Check sheet for the modelled part. Datum: model origin and axes. Units: mm. Face numbers are marked on the shaded views. A direction names the side the tool comes from. Coordinates: 2 decimals unless noted, no trailing zeros. Write each loop counter-clockwise with the first axis right and the second up, starting at its lowest first coordinate (ties: lowest second). Pieces come first, ordered by that corner, then holes. Notation, with made-up numbers: M 82,-30 L 115,-30 A25 cw 115,-17 Z; hole C 24,8 d7. An arc over 180 degrees is marked long. Answer as CSV lines item,"result".
from build123d import *

# Parameters (mm, degrees)
EXTRUDE1_DEPTH      = 3.9
EXTRUDE1_DEPTH_BACK = 3.9
SKETCH2_W           = 4.5
SKETCH2_H           = 25.2
SKETCH2_W_2         = 29.65
SKETCH2_H_2         = 5.85
EXTRUDE2_DEPTH      = 3.5
CHAMFER1_SIZE       = 3
CHAMFER1_SIZE2      = 3.451105222
CHAMFER2_SIZE       = 2
CHAMFER2_SIZE2      = 3.464101615
CHAMFER3_SIZE       = 1
EXTRUDE3_REACH      = 40.849
SKETCH4_R           = 3
FILLET1_R           = 0.8
EXTRUDE4_REACH      = 40.849
SKETCH5_R           = 3


# Read off the part's stored shape, not the designer's step: Mirror1
with BuildPart() as part:
    # Sketch1 → Extrude1 (new, two sides: drawn at the far end of the back side and taken through both)
    with BuildSketch(Plane.XY.offset(-EXTRUDE1_DEPTH_BACK)):
        Polygon((0, 0), (0, 29.8), (-7.2, 29.8), (-7.2, -7.2), (23.8, -7.2), (23.8, 0), align=None)
    extrude(amount=EXTRUDE1_DEPTH + EXTRUDE1_DEPTH_BACK)

    # Sketch2 → Extrude2 (add)
    with BuildSketch(Plane.XY.offset(3.9)):
        with Locations((-3.6, 17.2)):
            Rectangle(SKETCH2_W, SKETCH2_H)
        with Locations((8.975, -4.275)):
            Rectangle(SKETCH2_W_2, SKETCH2_H_2)
    extrude(amount=EXTRUDE2_DEPTH)

    # Chamfer1
    chamfer1_edges = [part.edges().sort_by_distance(p)[0] for p in [
        (23.8, -4.275, 7.4),
        (-5.85, -4.275, 7.4),
    ]]
    chamfer1_side = [part.faces().sort_by_distance(p)[0] for p in [
        (8.975, -4.275, 7.4),
    ]]
    chamfer(chamfer1_edges, length=CHAMFER1_SIZE, length2=CHAMFER1_SIZE2, reference=chamfer1_side[0])

    # Chamfer2
    chamfer2_edges = [part.edges().sort_by_distance(p)[0] for p in [
        (8.975, -7.2, 7.4),
    ]]
    chamfer2_side = [part.faces().sort_by_distance(p)[0] for p in [
        (8.975, -4.275, 7.4),
    ]]
    chamfer(chamfer2_edges, length=CHAMFER2_SIZE, length2=CHAMFER2_SIZE2, reference=chamfer2_side[0])

    # Chamfer3
    chamfer3_edges = [part.edges().sort_by_distance(p)[0] for p in [
        (-3.6, 29.8, 7.4),
        (-1.35, 17.2, 7.4),
        (-3.6, 4.6, 7.4),
        (-5.85, 17.2, 7.4),
    ]]
    chamfer(chamfer3_edges, length=CHAMFER3_SIZE)

    # Mirror1: part across plane


with BuildPart() as part_1:
    add(part.part)
    add(part.part.mirror(Plane.XY))

    # Sketch4 → Extrude3 (cut, up to next)
    with BuildSketch(Plane(origin=(0, 0, 0), x_dir=(1, 0, 0), z_dir=(0, 1, 0)), mode=Mode.PRIVATE) as extrude3_sk1:
        with Locations(Location((12.8, 0, 0), (0, 0, 270))):
            Circle(SKETCH4_R)
    extrude3_tool1 = extrude(extrude3_sk1.sketch, amount=-EXTRUDE3_REACH, mode=Mode.PRIVATE) & part_1.part
    add(extrude3_tool1.solids().sort_by_distance((12.8, 0, 0))[0], mode=Mode.SUBTRACT)

    # Fillet1
    fillet1_edges = [part_1.edges().sort_by_distance(p)[0] for p in [
        (-7.2, 29.8, 0),
        (23.8, -7.2, 0),
        (23.8, 0, 0),
        (0, 29.8, 0),
    ]]
    fillet(fillet1_edges, radius=FILLET1_R)

    # Sketch5 → Extrude4 (cut, up to next)
    with BuildSketch(Plane(origin=(0, 0, 0), x_dir=(0, 0, -1), z_dir=(1, 0, 0)), mode=Mode.PRIVATE) as extrude4_sk1:
        with Locations(Location((0, 17.8, 0), (0, 0, 90))):
            Circle(SKETCH5_R)
    extrude4_tool1 = extrude(extrude4_sk1.sketch, amount=-EXTRUDE4_REACH, mode=Mode.PRIVATE) & part_1.part
    add(extrude4_tool1.solids().sort_by_distance((0, 17.8, 0))[0], mode=Mode.SUBTRACT)


solid = part_1.part
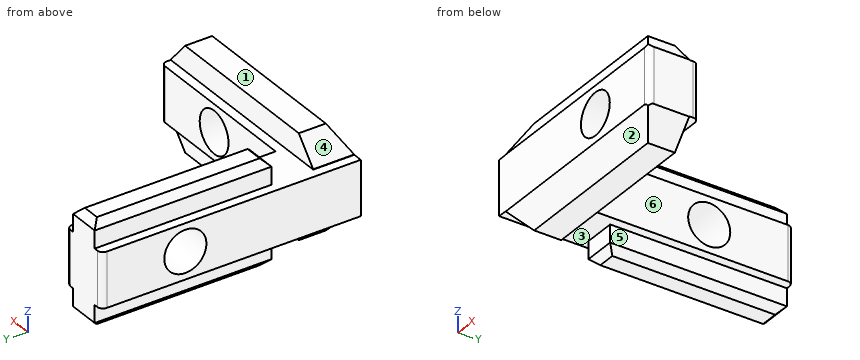
1) Thickness scan on line 1 along X through (y, z) = (-4.5, 0); line 2 along Z through (x, y) = (-3.75, 17.8); line 3 along Y through (x, z) = (22.5, 0.5). Record the ranges inside material, lowest first.
Answer key:
line 1,"x = -7.2 to 9.8, 15.8 to 23.8"
line 2,"z = -7.4 to -3, 3 to 7.4"
line 3,"y = -7.2 to 0"
2) Section check B-B, the plane y = 17.8. Record the boundary of the cut face in (x, z).
Answer key:
outline,"M -7.2,-3.9 L -5.85,-3.9 L -5.85,-6.4 L -4.85,-7.4 L -2.35,-7.4 L -1.35,-6.4 L -1.35,-3.9 L 0,-3.9 L 0,-3 L -7.2,-3 Z; M -7.2,3 L 0,3 L 0,3.9 L -1.35,3.9 L -1.35,6.4 L -2.35,7.4 L -4.85,7.4 L -5.85,6.4 L -5.85,3.9 L -7.2,3.9 Z"
3) Mould release check, pull along Y, two halves, no side actions. Record for the marked faces 1, 2 and 3: pulls with the +Y half, pulls with the -Y half, needs draft (parallel to the pull), parting line crosses it, or undercut.
Answer key:
face 1,"needs draft"
face 2,"pulls with the -Y half"
face 3,"undercut"
4) Tool access check on the marked faces 4, 5 and 6. Record the directions out of +Z, -Z, +X, -X, +Y, -Y that give a thin tool (end or side, any length) a straight path to the whole face; none if there is none.
Answer key:
face 4,"+Z, -X, -Y"
face 5,"-Z, +X, +Y"
face 6,"+Z, -Z, +X, +Y"
5) Section check D-D, the plane x = 8. Record the boundary of the cut face in (y, z), plus the area to 3 significant figures.
Answer key:
outline,"M -7.2,-3.94 L -5.2,-7.4 L -1.35,-7.4 L -1.35,-3.9 L 0,-3.9 L 0,3.9 L -1.35,3.9 L -1.35,7.4 L -5.2,7.4 L -7.2,3.94 Z"
area,"90.2 mm2"
6) Depth check by flat-ended pin: P1, Ø4, axis at x = 9, z = 6, coming from the +Y side; P2, Ø8, axis at x = 2.5, y = 7, coming from the +Z side; P3, Ø2, axis at y = 21, z = 5, coming from the +X side. Enter the tip coordinate at first touch or a pass-through.
Answer key:
P1,"stops at y = -1.35"
P2,"stops at z = 6.55"
P3,"stops at x = -1.35"
7) Section check C-C, the plane z = 0. Record the boundary of the cut face in (x, y), plus the area to 3 significant figures.
Answer key:
outline,"M -7.2,-7.2 L 9.8,-7.2 L 9.8,0 L 0,0 L 0,14.8 L -7.2,14.8 Z; M -7.2,20.8 L 0,20.8 L 0,29 A0.8 ccw -0.8,29.8 L -6.4,29.8 A0.8 ccw -7.2,29 Z; M 15.8,-7.2 L 23,-7.2 A0.8 ccw 23.8,-6.4 L 23.8,-0.8 A0.8 ccw 23,0 L 15.8,0 Z"
area,"351 mm2"
8) Section check A-A, the plane x = 12.8. Record the boundary of the cut face in (y, z), plus the area to 3 significant figures.
Answer key:
outline,"M -7.2,-3.94 L -5.2,-7.4 L -1.35,-7.4 L -1.35,-3.9 L 0,-3.9 L 0,-3 L -7.2,-3 Z; M -7.2,3 L 0,3 L 0,3.9 L -1.35,3.9 L -1.35,7.4 L -5.2,7.4 L -7.2,3.94 Z"
area,"47.0 mm2"
